The listing builds one solid part. Answer for the finished solid, in the listing's coordinates (mm). Face numbers are marked on the shaded views. A direction names the side the tool comes from. Give positions to 0.01 mm unless a question says otherwise; leave off trailing zeros. Loops run counter-clockwise (first coordinate to the right, second up) from the corner with the lowest first, then second, coordinate; pieces in that order, holes last. Notation, with made-up numbers: (4, 62) - (47, 62) arc R34 cw to (47, 93) - close; hole circle Ø5 at (61, 8). An arc over 180 degrees is marked (long way). Answer as CSV lines item,"result". Start each with the question number.
1) A cutting plane is placed at A-A (y = 5). Determine the outline of the cut face in (x, z).
2) A cutting plane is placed at B-B (x = -0.5). Determine the outline of the cut face in (y, z), and give its area (3 significant figures).
3) Flat-ended cylindrical pins translate along their axes: pin 1 (1.4 mm diameter, centred on x = 5.97, z = 20.98, fed in from -Y); pin 2 (20 mm diameter, centred on x = -1, y = -1, fed in from +Z); pin 3 (4 mm diameter, centred on x = -7.5, y = -12.5, fed in from +Z). Find the tip coordinate at first contact, or state that the pin passes through.
4) For the marked faces 5 and 6, determine the directions among +Z, -Z, +X, -X, +Y, -Y from which every point of the face is accessible in a straight line to the end or side of a thin tool.
5) A cutting plane is placed at C-C (y = -13.5). Determine the outline of the cut face in (x, z), and give its area (3 significant figures).
6) A cutting plane is placed at D-D (y = 9.5). Determine the outline of the cut face in (x, z), and give its area (3 significant figures).
7) For a pull along Y with two mould halves and no side action, classify the marked faces 1, 2, 3 and 4 as pulls with the +Y half, pulls with the -Y half, needs draft (parallel to the pull), parting line crosses it, or undercut.
8) Find the intervals of material crossed by line 1 along Y through (x, z) = (3.5, 9); line 2 along Y through (x, z) = (4, 22); line 3 along X through (y, z) = (15.7, 27), in increasing order.
```python
from build123d import *

# Parameters (mm, degrees)
ESBO_O1_W                  = 40
ESBO_O1_H                  = 34
ESBO_O1_R                  = 1.5
ESBO_O1_W_2                = 22.5
ESBO_O1_H_2                = 12
RESSALTO_EXTRUS_O1_DEPTH   = 3
ESBO_O2_W                  = 40
ESBO_O2_H                  = 2.5
RESSALTO_EXTRUS_O2_DEPTH   = 30
CORTE_EXTRUS_O1_DEPTH      = 53.282720471
CORTE_EXTRUS_O1_DEPTH_BACK = 53.282720471
ESBO_O3_R                  = 3.5
FILETE1_R                  = 6
FILETE2_R                  = 2
CORTE_EXTRUS_O2_DEPTH      = 1
FILETE4_R                  = 8
CORTE_EXTRUS_O3_REACH      = 53.638
ESBO_O5_R                  = 0.6


with BuildPart() as part:
    # Esboço1 → Ressalto-extrusão1 (new body)
    with BuildSketch(Plane.XY):
        with Locations((-2.101648352, 0.459478022)):
            Rectangle(ESBO_O1_W, ESBO_O1_H)
        with Locations((11.648351648, 0.459478022)):
            Circle(ESBO_O1_R, mode=Mode.SUBTRACT)
        with Locations(Location((-15.851648352, 0.459478022, 0), (0, 0, 180))):
            Circle(ESBO_O1_R, mode=Mode.SUBTRACT)
        with Locations((-2.101648352, 0.459478022)):
            Rectangle(ESBO_O1_W_2, ESBO_O1_H_2, mode=Mode.SUBTRACT)
    extrude(amount=RESSALTO_EXTRUS_O1_DEPTH)

    # Esboço2 → Ressalto-extrusão2 (add)
    with BuildSketch(Plane.XY.offset(3)):
        with Locations((-2.101648352, 16.209478022)):
            Rectangle(ESBO_O2_W, ESBO_O2_H)
        with Locations((-2.101648352, -15.290521978)):
            Rectangle(ESBO_O2_W, ESBO_O2_H)
    extrude(amount=RESSALTO_EXTRUS_O2_DEPTH)

    # Esboço3 → Corte-extrusão1 (cut, two sides: drawn at the far end of the back side and taken through both)
    with BuildSketch(Plane.XZ.offset(16.540521978).offset(-CORTE_EXTRUS_O1_DEPTH_BACK)):
        with Locations(Location((11.898351648, 27, 0), (0, 0, 270))):
            Circle(ESBO_O3_R)
        Polygon((-22.101648352, 3), (7.898351648, 33), (-22.101648352, 33), align=None)
    extrude(amount=CORTE_EXTRUS_O1_DEPTH + CORTE_EXTRUS_O1_DEPTH_BACK, mode=Mode.SUBTRACT)

    # Filete1
    filete1_edges = [part.edges().sort_by_distance(p)[0] for p in [
        (17.898351648, 16.209478022, 33),
        (17.898351648, -15.290521978, 33),
    ]]
    fillet(filete1_edges, radius=FILETE1_R)

    # Filete2
    filete2_edges = [part.edges().sort_by_distance(p)[0] for p in [
        (-2.101648352, 14.959478022, 3),
        (-2.101648352, -14.040521978, 3),
    ]]
    fillet(filete2_edges, radius=FILETE2_R)

    # Esboço4 → Corte-extrusão2 (cut)
    with BuildSketch(Plane.XZ.offset(16.540521978)):
        with BuildLine():
            Line((5.173317787, 23.74427083), (-1.45414508, 17.053728929))
            Line((-1.45414508, 17.053728929), (1.905973753, 13.7252896))
            Line((1.905973753, 13.7252896), (8.413154378, 20.294404433))
            ThreePointArc((8.413154378, 20.294404433), (9.16091607, 20.97650137), (9.973796219, 21.579518488))
            Line((9.973796219, 21.579518488), (13.290279513, 23.788686123))
            Line((13.290279513, 23.788686123), (11.68978022, 23.506220104))
            Line((11.68978022, 23.506220104), (8.398351648, 27))
            Line((8.398351648, 27), (8.903771348, 28.811764009))
            Line((8.903771348, 28.811764009), (6.253622951, 25.036396208))
            ThreePointArc((6.253622951, 25.036396208), (5.740721803, 24.367549457), (5.173317787, 23.74427083))
        make_face()
    extrude(amount=-CORTE_EXTRUS_O2_DEPTH, mode=Mode.SUBTRACT)

    # Filete4
    filete4_edges = [part.edges().sort_by_distance(p)[0] for p in [
        (7.898351648, -15.290521978, 33),
        (7.898351648, 16.209478022, 33),
    ]]
    fillet(filete4_edges, radius=FILETE4_R)

    # Esboço5 → Corte-extrusão3 (cut, up to next)
    with BuildSketch(Plane(origin=(0, -15.540521978, 0), x_dir=(-1, 0, 0), z_dir=(0, -1, 0)), mode=Mode.PRIVATE) as corte_extrus_o3_sk1:
        with Locations(Location((-8.774251962, -23.831009443, 0), (0, 0, 180))):
            Circle(ESBO_O5_R)
    corte_extrus_o3_tool1 = extrude(corte_extrus_o3_sk1.sketch, amount=-CORTE_EXTRUS_O3_REACH, mode=Mode.PRIVATE) & part.part
    # Esboço5 → Corte-extrusão3 (cut, up to next)
    with BuildSketch(Plane(origin=(0, -15.540521978, 0), x_dir=(-1, 0, 0), z_dir=(0, -1, 0)), mode=Mode.PRIVATE) as corte_extrus_o3_sk2:
        with Locations(Location((-5.966072468, -20.982478606, 0), (0, 0, 180))):
            Circle(ESBO_O5_R)
    corte_extrus_o3_tool2 = extrude(corte_extrus_o3_sk2.sketch, amount=-CORTE_EXTRUS_O3_REACH, mode=Mode.PRIVATE) & part.part
    # Esboço5 → Corte-extrusão3 (cut, up to next)
    with BuildSketch(Plane(origin=(0, -15.540521978, 0), x_dir=(-1, 0, 0), z_dir=(0, -1, 0)), mode=Mode.PRIVATE) as corte_extrus_o3_sk3:
        with Locations(Location((-1.753803228, -16.70968235, 0), (0, 0, 180))):
            Circle(ESBO_O5_R)
    corte_extrus_o3_tool3 = extrude(corte_extrus_o3_sk3.sketch, amount=-CORTE_EXTRUS_O3_REACH, mode=Mode.PRIVATE) & part.part
    add(corte_extrus_o3_tool1.solids().sort_by_distance((8.774252, -15.540522, 23.831009))[0], mode=Mode.SUBTRACT)
    add(corte_extrus_o3_tool2.solids().sort_by_distance((5.966072, -15.540522, 20.982479))[0], mode=Mode.SUBTRACT)
    add(corte_extrus_o3_tool3.solids().sort_by_distance((1.753803, -15.540522, 16.709682))[0], mode=Mode.SUBTRACT)


solid = part.part
```
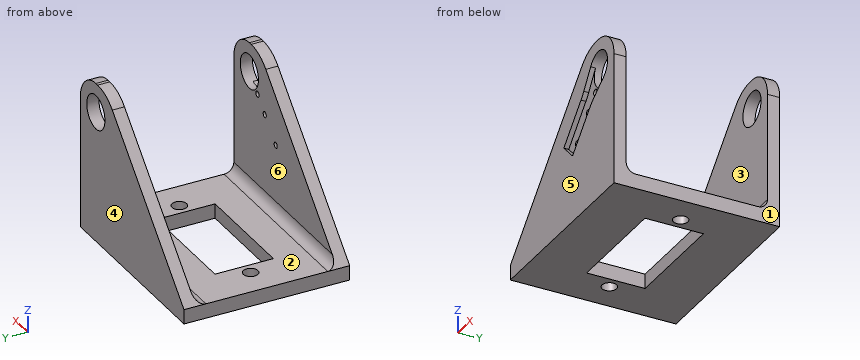
Ans:
1,outline,"(-22.1, 0) - (-13.35, 0) - (-13.35, 3) - (-22.1, 3) - close; (9.15, 0) - (17.9, 0) - (17.9, 3) - (9.15, 3) - close"
2,outline,"(-16.54, 0) - (-5.54, 0) - (-5.54, 3) - (-12.04, 3) arc R2 cw to (-14.04, 5) - (-14.04, 24.6) - (-16.54, 24.6) - (-16.54, 18.02) - (-15.54, 18.02) - (-15.54, 16.11) - (-16.54, 16.11) - close; (6.46, 0) - (17.46, 0) - (17.46, 24.6) - (14.96, 24.6) - (14.96, 5) arc R2 cw to (12.96, 3) - (6.46, 3) - close"
2,area,"174 mm2"
3,pin 1,"y = -15.54"
3,pin 2,"z = 3"
3,pin 3,"z = 18.88"
4,face 5,"+Z, -Z, +X, -X, -Y"
4,face 6,"+Z, +X, -X"
5,outline,"(-22.1, 0) - (17.9, 0) - (17.9, 3.63) - (-21.47, 3.63) - (-22.1, 3) - close"
5,area,"145 mm2"
6,outline,"(-22.1, 0) - (17.9, 0) - (17.9, 3) - (-22.1, 3) - close"
6,area,"120 mm2"
7,face 1,"needs draft"
7,face 2,"undercut"
7,face 3,"undercut"
7,face 4,"pulls with the +Y half"
8,line 1,"-16.54 to -14.04, 14.96 to 17.46"
8,line 2,"-15.54 to -14.04, 14.96 to 17.46"
8,line 3,"1.9 to 8.4, 15.4 to 17.9"
